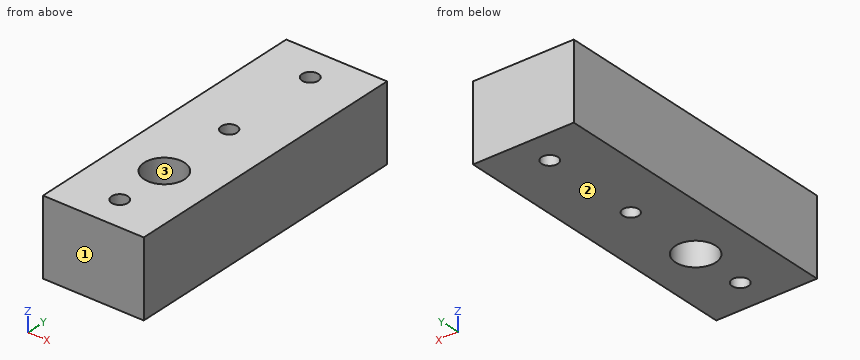
Autodesk Inventor part; units mm, degrees
ref_plane "YZ Plane" through (0, 0, 0) normal (1, 0, 0) x (0, 1, 0)
ref_plane "XZ Plane" through (0, 0, 0) normal (0, 1, 0) x (-1, 0, 0)
ref_plane "XY Plane" through (0, 0, 0) normal (0, 0, 1) x (1, 0, 0)
sketch "스케치1" plane through (0, 0, 0) normal (0, 0, 1) x (1, 0, 0)
  line L0 (0, 0) -> (4, 0)
  line L1 (4, 0) -> (4, 12)
  line L2 (4, 12) -> (0, 12)
  line L3 (0, 12) -> (0, 0)
  dimension "d0" = 4
  dimension "d1" = 12
extrude "돌출1" add sketch "스케치1" along normal blind 3
sketch "스케치2" plane through (0, 0, 3) normal (0, 0, 1) x (1, 0, 0)
  line L0 (4, 12) -> (0, 12) construction
  line L1 (2, 12) -> (2, 0) construction
  line L2 (0, 0) -> (4, 0) construction
  line L3 (4, 0) -> (4, 12)
  line L4 (0, 12) -> (0, 0)
  point P0 (2, 6.7)
  point P1 (2, 3.5)
  point P2 (2, 1.3)
  point P3 (2, 10.7)
  dimension "d45" = 1.3
  dimension "d52" = 2.2
  dimension "d55" = 1.3
  dimension "d57" = 3.2
hole "구멍1" at (2, 6.7, 3) direction (0, 0, -1) diameter 0.63 end through all
hole "구멍2" at (2, 3.5, 3) direction (0, 0, -1) diameter 1.6 end through all
hole "구멍3" at (2, 1.3, 3) at (2, 10.7, 3) direction (0, 0, -1) diameter 0.65 end through all
equation "\"G23_M\" = 0.67"
equation "\"G23_F\" = 0.65"
properties part number "Top" material "유리"
Build history of the part. All positions in model axes, mm. Face numbers are marked on the shaded views. Give positions to 0.01 mm unless a question says otherwise; leave off trailing zeros. Order: outer loops, then holes, each group sorted by start corner. A loop starts at its lowest first (then second) coordinate and runs counter-clockwise, first axis right, second up. Notation, with made-up numbers: M -38.75,-10.75 L -20.75,-10.75 A16 cw -20.75,-2.75 Z; hole C 88.25,47 d7. An arc over 180 degrees is marked long. Write item = value, one per line. Start each with the question number.
(1) Slice it at B-B on x = 2. Write the cut outline in (y, z) (3 decimals), plus the area to 3 significant figures.
(2) Slice it at C-C on z = 0.3. Write the cut outline in (x, y) (3 decimals), plus the area to 3 significant figures.
(3) Slice it at D-D on y = 1.3. Write the cut outline in (x, z) (3 decimals), plus the area to 4 significant figures.
(4) Slice it at A-A on y = 6.7. Write the cut outline in (x, z) (3 decimals), plus the area to 3 significant figures.
(5) Two-plate mould, pull along Y, no slides. Class the marked faces 1, 2 and 3: released by +Y, released by -Y, zero draft, split by the parting line, or undercut.
(6) Probe L1, parallel to Y at x = 2, z = 2.2 (3 decimals); L2, parallel to X at y = 10.7, z = 2.1 (3 decimals); L3, parallel to Y at x = 1.45, z = 1.65. List the from-to ranges inside material, lowest first. Write a range as [from, to].
Responses:
q1.outline = M 0,0 L 0.975,0 L 0.975,3 L 0,3 Z; M 1.625,0 L 2.7,0 L 2.7,3 L 1.625,3 Z; M 4.3,0 L 6.385,0 L 6.385,3 L 4.3,3 Z; M 7.015,0 L 10.375,0 L 10.375,3 L 7.015,3 Z; M 11.025,0 L 12,0 L 12,3 L 11.025,3 Z
q1.area = 25.4 mm2
q2.outline = M 0,0 L 4,0 L 4,12 L 0,12 Z; hole C 2,3.5 d1.6; hole C 2,1.3 d0.65; hole C 2,10.7 d0.65; hole C 2,6.7 d0.63
q2.area = 45.0 mm2
q3.outline = M 0,0 L 1.675,0 L 1.675,3 L 0,3 Z; M 2.325,0 L 4,0 L 4,3 L 2.325,3 Z
q3.area = 10.05 mm2
q4.outline = M 0,0 L 1.685,0 L 1.685,3 L 0,3 Z; M 2.315,0 L 4,0 L 4,3 L 2.315,3 Z
q4.area = 10.1 mm2
q5.face_1 = released by -Y
q5.face_2 = zero draft
q5.face_3 = undercut
q6.L1 = [0, 0.975], [1.625, 2.7], [4.3, 6.385], [7.015, 10.375], [11.025, 12]
q6.L2 = [0, 1.675], [2.325, 4]
q6.L3 = [0, 2.92], [4.08, 12]
